Geometry check sheet. Reference: the model listing, model coordinates, mm. A direction names the side the tool comes from. Give positions to 0.01 mm unless a question says otherwise; leave off trailing zeros. Order: outer loops, then holes, each group sorted by start corner. A loop starts at its lowest first (then second) coordinate and runs counter-clockwise, first axis right, second up. Notation, with made-up numbers: (42, 3) - (91, 3) arc R16 ccw to (91, 23) - close; hole circle Ø3 at (-39.5, 56). An arc over 180 degrees is marked (long way). Put each result on its own line as item: value. Start each with the question number.
```python
from build123d import *

# Parameters (mm, degrees)
F0_W     = 87
F0_H     = 78
F0_W_2   = 62.5
F0_H_2   = 66
F1_DEPTH = 37
F2_DEPTH = 77
F3_ANGLE = 90


with BuildPart() as f1:
    # F0 (on Top) → F1 (new body)
    with BuildSketch(Plane.XY):
        with Locations((-1.143673, 10.111042)):
            Rectangle(F0_W, F0_H)
        with Locations((-1.143673, 7.111042)):
            Rectangle(F0_W_2, F0_H_2, mode=Mode.SUBTRACT)
        with Locations((-1.143673, 7.111042)):
            Rectangle(F0_W_2, F0_H_2)
    extrude(amount=F1_DEPTH)

    # F0 (on Top) → F2 (join)
    with BuildSketch(Plane.XY):
        with Locations((-1.143673, 7.111042)):
            Rectangle(F0_W_2, F0_H_2)
    extrude(amount=-F2_DEPTH)


with BuildPart() as f1_1:
    # F3: moved
    add(f1.part.rotate(Axis((-32.393673, -25.888958, -38.5), (0, 0, 1)), F3_ANGLE))


solid = f1_1.part
```
Item 1: Set-up check for faces 1 (the face through (-32.394, 5, -38)), 2 (the face through (-65, 36.611, -38)), 3 (the face through (-98.394, 5, -38)), 4 (the face through (-65, -25.889, -38)): record each of +Z, -Z, +X, -X, +Y, -Y from which the full face is reachable in a straight line by a thin tool's end or side.
Item 2: Cross-section at B-B (x = -46.5). Enter the section's corners in (y, z).
Item 3: Gauge pin test, flat ends, axial feed: pin 1 Ø5 at (y, z) = (11.5, -60) entering from -X; pin 2 Ø1 at (x, z) = (-97.5, -37.5) entering from -Y. Record the tip position at first contact, or that the pin passes through.
Item 4: Cross-section at A-A (y = 25.5). Enter the section's corners in (x, z), and give its area (3 significant figures).
Item 5: Cross-section at C-C (z = -9). Enter the section's corners in (x, y), and give its area (4 significant figures).
Item 6: Thickness scan on line 1 along Z through (x, y) = (-52, 45); line 2 along X through (y, z) = (17, -56.5); line 3 along Y through (x, z) = (-40, -40). Record the ranges inside material, lowest first.
Item 7: Cross-section at D-D (y = 40). Enter the section's corners in (x, z).
Recorded:
1. face 1: -Z, +X, +Y, -Y
1. face 2: -Z, +X, -X, +Y
1. face 3: -Z, -X, +Y, -Y
1. face 4: -Z, +X, -X, -Y
2. outline: (-38.14, 0) - (-25.89, 0) - (-25.89, -77) - (36.61, -77) - (36.61, 0) - (48.86, 0) - (48.86, 37) - (-38.14, 37) - close
3. pin 1: stops at x = -98.39
3. pin 2: stops at y = -25.89
4. outline: (-107.39, 0) - (-98.39, 0) - (-98.39, -77) - (-32.39, -77) - (-32.39, 0) - (-29.39, 0) - (-29.39, 37) - (-107.39, 37) - close
4. area: 7,970 mm^2
5. outline: (-98.39, -25.89) - (-32.39, -25.89) - (-32.39, 36.61) - (-98.39, 36.61) - close
5. area: 4,125 mm^2
6. line 1: z = 0 to 37
6. line 2: x = -98.39 to -32.39
6. line 3: y = -25.89 to 36.61
7. outline: (-107.39, 0) - (-29.39, 0) - (-29.39, 37) - (-107.39, 37) - close
